Geometry check sheet. Reference: the model listing, model coordinates, mm. Round coordinates to 2 decimals unless told otherwise and drop trailing zeros. Order: outer loops, then holes, each group sorted by start corner. A loop starts at its lowest first (then second) coordinate and runs counter-clockwise, first axis right, second up. Notation, with made-up numbers: (-33.5, -18) - (-22.5, -18) arc R20 cw to (-22.5, -14) - close; hole circle Ø3 at (16.5, 80.5). An arc over 180 degrees is marked (long way). Return JSON: item names as keys, results as strings. Group by question number.
Q1. Sectioned sample at A-A, the plane z = 2.05. Record the cut outline in (x, y), then the cut area to 3 significant figures.
Q2. Material ranges on line 1 along X through (y, z) = (37, 0.25); line 2 along Y through (x, z) = (57, 0.75); line 3 along X through (y, z) = (47.5, 1.3), recorded low to high.
Q3. Gauge pin test, flat ends, axial feed: pin 1 Ø1 at (y, z) = (53, 1) entering from +X; pin 2 Ø1.5 at (y, z) = (19, 1.5) entering from +X. Record the tip position at first contact, or that the pin passes through.
Q4. Sectioned sample at B-B, the plane y = 27. Record the cut outline in (x, z).
Q5. Sectioned sample at C-C, the plane x = 68. Record the cut outline in (y, z), then the cut area to 3 significant figures.
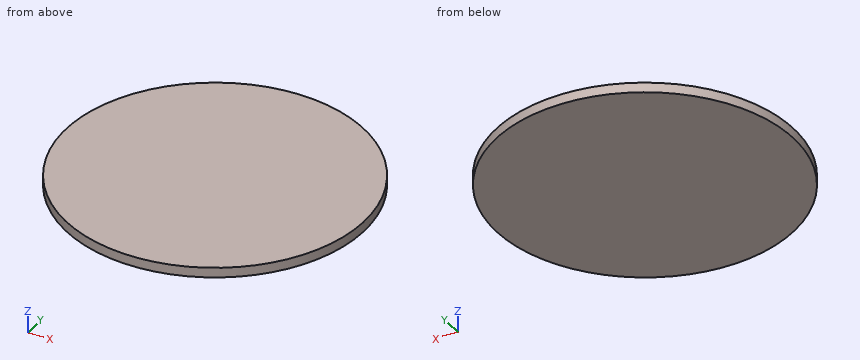
Autodesk Fusion 360 part; units mm, degrees
cylinder "CylinderPrimitive1" add diameter 76.2 height 2.54 placed x (1, 0, 0) y (0, 1, 0) z (0, 0, 1) at (40.64, 38.1, 0) in component "Disk"
component "Disk" placed x (1, 0, 0) y (0, 1, 0) z (0, 0, 1) at (0, 0, 0)
component "Component" placed x (1, 0, 0) y (0, 1, 0) z (0, 0, 1) at (0, 0, 0)
Reply:
{
 "1": {"outline": "circle Ø76.2 at (40.64, 38.1)", "area": "4,560 mm^2"},
 "2": {"line 1": "2.56 to 78.72", "line 2": "3.69 to 72.51", "line 3": "3.72 to 77.56"},
 "3": {"pin 1": "x = 75.91", "pin 2": "x = 74.03"},
 "4": {"outline": "(4.19, 0) - (77.09, 0) - (77.09, 2.54) - (4.19, 2.54) - close"},
 "5": {"outline": "(11.59, 0) - (64.61, 0) - (64.61, 2.54) - (11.59, 2.54) - close", "area": "135 mm^2"}
}
